```python
from build123d import *

# Parameters (mm, degrees)
SKETCH1_R                = 3
SKETCH1_R_2              = 1.5
SKETCH1_W                = 2
SKETCH1_H                = 12
SKETCH1_W_2              = 12
SKETCH1_H_2              = 22.5
SKETCH1_W_3              = 12.5
SKETCH1_H_3              = 23
BOSS_EXTRUDE2_DEPTH      = 2
F_3_0_3_DIAMETER_HOLE1_D = 3
F_3_0_3_DIAMETER_HOLE2_D = 3


with BuildPart() as part:
    # Sketch1 → Boss-Extrude2 (new body)
    with BuildSketch(Plane(origin=(0, 0, 0), x_dir=(1, 0, 0), z_dir=(0, 1, 0))):
        with BuildLine():
            Line((47.026548113, 113.484810936), (-47.026548113, 113.484810936))
            ThreePointArc((-47.026548113, 113.484810936), (-54.774215022, 112.467109973), (-61.996228059, 109.483054768))
            Line((-61.996228059, 109.483054768), (-87, 95.085987572))
            Line((-87, 95.085987572), (-87, 85.085987572))
            Line((-87, 85.085987572), (-77, 85.085987572))
            Line((-77, 85.085987572), (-77, 91.313276712))
            Line((-77, 91.313276712), (-63.105457223, 99.313696268))
            Line((-63.105457223, 99.313696268), (-63.105457223, 88.484810936))
            Line((-63.105457223, 88.484810936), (-37.5, 88.484810936))
            Line((-37.5, 88.484810936), (-37.5, 48.484810936))
            Line((-37.5, 48.484810936), (-52.5, 48.484810936))
            Line((-52.5, 48.484810936), (-52.5, 28.484810936))
            Line((-52.5, 28.484810936), (-37.5, 28.484810936))
            Line((-37.5, 28.484810936), (-37.5, -11.515189064))
            Line((-37.5, -11.515189064), (-87, -11.515189064))
            Line((-87, -11.515189064), (-87, -199.484504535))
            Line((-87, -199.484504535), (-59.5, -199.484504535))
            Line((-59.5, -199.484504535), (-59.5, -274.484504535))
            Line((-59.5, -274.484504535), (-87, -274.484504535))
            Line((-87, -274.484504535), (-87, -275.742175661))
            Line((-87, -275.742175661), (-87, -285.742175661))
            Line((-87, -285.742175661), (-50.740945714, -315.558389864))
            Line((-50.740945714, -315.558389864), (50.740945714, -315.558389864))
            Line((50.740945714, -315.558389864), (87, -285.742175661))
            Line((87, -285.742175661), (87, -275.742175661))
            Line((87, -275.742175661), (87, -274.484504535))
            Line((87, -274.484504535), (59.5, -274.484504535))
            Line((59.5, -274.484504535), (59.5, -199.484504535))
            Line((59.5, -199.484504535), (87, -199.484504535))
            Line((87, -199.484504535), (87, -11.515189064))
            Line((87, -11.515189064), (37.5, -11.515189064))
            Line((37.5, -11.515189064), (37.5, 28.484810936))
            Line((37.5, 28.484810936), (52.5, 28.484810936))
            Line((52.5, 28.484810936), (52.5, 48.484810936))
            Line((52.5, 48.484810936), (37.5, 48.484810936))
            Line((37.5, 48.484810936), (37.5, 88.484810936))
            Line((37.5, 88.484810936), (63.105457223, 88.484810936))
            Line((63.105457223, 88.484810936), (63.105457223, 99.313696268))
            Line((63.105457223, 99.313696268), (77, 91.313276712))
            Line((77, 91.313276712), (77, 85.085987572))
            Line((77, 85.085987572), (87, 85.085987572))
            Line((87, 85.085987572), (87, 95.085987572))
            Line((87, 95.085987572), (61.996228059, 109.483054768))
            ThreePointArc((61.996228059, 109.483054768), (54.774215022, 112.467109973), (47.026548113, 113.484810936))
        make_face()
        with Locations(Location((-45, 38.484810936, 0), (0, 0, 270))):
            Circle(SKETCH1_R, mode=Mode.SUBTRACT)
        with Locations(Location((45, 38.484810936, 0), (0, 0, 90))):
            Circle(SKETCH1_R, mode=Mode.SUBTRACT)
        with Locations(Location((0, 38.804810936, 0), (0, 0, 270))):
            Circle(SKETCH1_R_2, mode=Mode.SUBTRACT)
        with Locations(Location((0, 66.104810936, 0), (0, 0, 90))):
            Circle(SKETCH1_R_2, mode=Mode.SUBTRACT)
        with Locations(Location((0, 79.56209058, 0), (0, 0, 270))):
            Circle(SKETCH1_R_2, mode=Mode.SUBTRACT)
        with Locations(Location((0, 106.86209058, 0), (0, 0, 90))):
            Circle(SKETCH1_R_2, mode=Mode.SUBTRACT)
        with Locations((-33.5, -258.484504535)):
            Rectangle(SKETCH1_W, SKETCH1_H, mode=Mode.SUBTRACT)
        with Locations((-56.5, -258.484504535)):
            Rectangle(SKETCH1_W, SKETCH1_H, mode=Mode.SUBTRACT)
        with Locations((-33.5, -210.484504535)):
            Rectangle(SKETCH1_W, SKETCH1_H, mode=Mode.SUBTRACT)
        with Locations((-56.5, -210.484504535)):
            Rectangle(SKETCH1_W, SKETCH1_H, mode=Mode.SUBTRACT)
        with Locations((56.5, -210.484504535)):
            Rectangle(SKETCH1_W, SKETCH1_H, mode=Mode.SUBTRACT)
        with Locations((33.5, -210.484504535)):
            Rectangle(SKETCH1_W, SKETCH1_H, mode=Mode.SUBTRACT)
        with Locations((56.5, -258.484504535)):
            Rectangle(SKETCH1_W, SKETCH1_H, mode=Mode.SUBTRACT)
        with Locations((33.5, -258.484504535)):
            Rectangle(SKETCH1_W, SKETCH1_H, mode=Mode.SUBTRACT)
        with Locations((0, 52.454810936)):
            Rectangle(SKETCH1_W_2, SKETCH1_H_2, mode=Mode.SUBTRACT)
        with Locations((0, 93.21209058)):
            Rectangle(SKETCH1_W_3, SKETCH1_H_3, mode=Mode.SUBTRACT)
    extrude(amount=BOSS_EXTRUDE2_DEPTH)

    # Ø3.0 (3) Diameter Hole1 (through all)
    with Locations(Plane(origin=(-77.532035134, 2, -197.100991793), x_dir=(1, 0, 0), z_dir=(0, 1, 0))):
        with Locations((97.86378973, -199.745008939), (69.96378973, -199.745008939), (54.76378973, -250.545008939), (102.56378973, -251.645008939)):
            Hole(F_3_0_3_DIAMETER_HOLE1_D / 2)

    # Ø3.0 (3) Diameter Hole2 (through all)
    with Locations(Plane(origin=(-77.532035134, 4, -197.100991793), x_dir=(1, 0, 0), z_dir=(0, 1, 0))):
        with Locations((97.918849389, -293.673103718), (58.918849389, -293.673103718), (58.918849389, -332.673103718), (97.918849389, -332.673103718)):
            Hole(F_3_0_3_DIAMETER_HOLE2_D / 2)


solid = part.part
```
Build history of the part. All positions in model axes, mm. A direction names the side the tool comes from. Round coordinates to 2 decimals unless told otherwise and drop trailing zeros. Loops run counter-clockwise (first coordinate to the right, second up) from the corner with the lowest first, then second, coordinate; pieces in that order, holes last.
Item 1: Two-plate mould, pull along X, no slides. Class faces 3 (the face through (-69.124, 0.986, 300.442)), 4 (the face through (69.955, 0.986, -95.369)), 5 (the face through (68.617, 0.986, 300.859)): released by +X, released by -X, zero draft, split by the parting line, or undercut.
Item 2: Drill centre lines: line 1 along Z through (x, y) = (49, 0.1); line 2 along X through (y, z) = (1.75, -84.5); line 3 along Z through (x, y) = (-23, 1.65). Where is each one in solid material? Low to high.
Item 3: Saw through at C-C (y = 1.2). State how many separate pieces and enclosed holes the cut face has, then the cut area to 3 significant figures.
Item 4: Which spindle directions (+Z, -Z, +X, -X, +Y, -Y) get a long thin tool onto all of the face, cutting with end or side? Do faces 1 (the face through (-1, 0, 98)), 2 (the face through (-70.15, 0.986, -95.257)). Say none if no direction does.
Item 5: Saw through at B-B (z = -17.5). List the corners of the cut face in (x, y).
Item 6: Saw through at A-A (z = 260). List the corners of the cut face in (x, y).
Item 7: Pin check, flat tips, straight feed: P1, Ø1, axis at y = 0.5, z = 257, coming from the +X side; P2, Ø3.5, axis at x = -45, z = -38.48, coming from the +Y side; P3, Ø0.6, axis at y = 1, z = -7.5, coming from the -X side; P4, Ø1, axis at y = 0.5, z = -37.5, coming from the +X side. Stop position of each tip, or through.
Worked answers:
1. face 3: released by -X
1. face 4: undercut
1. face 5: released by +X
2. line 1: z = -113.42 to -88.48, -48.48 to -28.48, 11.52 to 315.56
2. line 2: x = -37.5 to -6.25, 6.25 to 37.5
2. line 3: z = -113.48 to 51.96, 54.93 to 315.56
3. separate pieces: 1
3. enclosed holes: 24
3. area: 58,500 mm2
4. face 1: +Z, -Z, +X, -X, -Y
4. face 2: +Y, -Y
5. outline: (-37.5, 0) - (37.5, 0) - (37.5, 2) - (-37.5, 2) - close
6. outline: (-59.5, 0) - (-57.5, 0) - (-57.5, 2) - (-59.5, 2) - close; (-55.5, 0) - (-34.5, 0) - (-34.5, 2) - (-55.5, 2) - close; (-32.5, 0) - (32.5, 0) - (32.5, 2) - (-32.5, 2) - close; (34.5, 0) - (55.5, 0) - (55.5, 2) - (34.5, 2) - close; (57.5, 0) - (59.5, 0) - (59.5, 2) - (57.5, 2) - close
7. P1: stops at x = 59.5
7. P2: passes through
7. P3: stops at x = -37.5
7. P4: stops at x = 52.5
